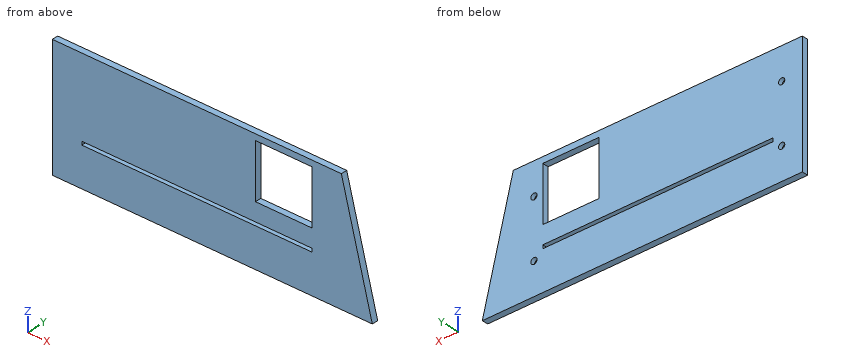
from build123d import *

# Parameters (mm, degrees)
F0_W     = 140
F0_H     = 59
F1_DEPTH = 3
F2_W     = 111.440674
F2_H     = 1.685995
F3_DEPTH = 25
F4_W     = 27.34
F4_H     = 19
F5_DEPTH = 25
F6_R     = 1.5
F7_DEPTH = 2
F8_W     = 27.34
F8_H     = 26.557377
F9_DEPTH = 25


with BuildPart() as f1:
    # F0 (on Front) → F1 (new body)
    with BuildSketch(Plane.XZ):
        Rectangle(F0_W, F0_H)
        Polygon((85, -29.5), (70, 29.5), (70, -29.5), align=None)
    extrude(amount=F1_DEPTH)

    # F2 (on face) → F3 (cut)
    with BuildSketch(Plane.XZ.offset(3)):
        with Locations((0, -9.62422)):
            Rectangle(F2_W, F2_H)
    extrude(amount=-F3_DEPTH, mode=Mode.SUBTRACT)

    # F4 (on face) → F5 (cut)
    with BuildSketch(Plane.XZ.offset(3)):
        with Locations((42.050337, 12.718777)):
            Rectangle(F4_W, F4_H)
    extrude(amount=-F5_DEPTH, mode=Mode.SUBTRACT)

    # F6 (on face) → F7 (cut)
    with BuildSketch(Plane(origin=(0, 0, 0), x_dir=(-1, 0, 0), z_dir=(0, 1, 0))):
        with Locations((60, 14)):
            Circle(F6_R)
        with Locations((-60, 14)):
            Circle(F6_R)
        with Locations((60, -14)):
            Circle(F6_R)
        with Locations((-60, -14)):
            Circle(F6_R)
    extrude(amount=-F7_DEPTH, mode=Mode.SUBTRACT)

    # F8 (on face) → F9 (cut)
    with BuildSketch(Plane.XZ.offset(3)):
        with Locations((42.050337, 13.278688)):
            Rectangle(F8_W, F8_H)
    extrude(amount=-F9_DEPTH, mode=Mode.SUBTRACT)


solid = f1.part
Source: CAD feature listing. Evaluate the final solid. Frame: model axes, mm. Round coordinates to 2 decimals unless told otherwise and drop trailing zeros. Order: outer loops, then holes, each group sorted by start corner. A loop starts at its lowest first (then second) coordinate and runs counter-clockwise, first axis right, second up. Notation, with made-up numbers: (26.25, 33.25) - (59.25, 33.25) arc R27 ccw to (59.25, 69.25) - close; hole circle Ø4 at (17, -13). An arc over 180 degrees is marked (long way). Use a Markdown table: item, result. Add a question column.
1. Section query A-A (x = 39). Return the cut outline in (y, z).
2. Section query D-D (z = 14). Return the cut outline in (x, y).
3. Line query: probe 1 along Z at (x, y) = (60, -0.5); probe 2 along Z at (x, y) = (34, -2.1); probe 3 along Z at (x, y) = (13, -2.45). Output: solid intervals per line, ascending.
4. Section query C-C (x = -32). Return the cut outline in (y, z), then the cut area to 3 significant figures.
5. First-contact query: pin 1 (5 mm diameter, centred on x = 1, z = -18.5, fed in from +Y); pin 2 (0.5 mm diameter, centred on y = -2, z = -9.5, fed in from +X); pin 3 (1.5 mm diameter, centred on y = -2, z = 8.5, fed in from +X); pin 4 (0.9 mm diameter, centred on x = -60.5, z = -14.5, fed in from +Y). Flat tips, straight axial feed; report the tip coordinate or a pass-through.
6. Section query B-B (y = -0.85). Return the cut outline in (x, z).
Derived:
| question | item | result |
|---|---|---|
| 1 | outline | (-3, -29.5) - (0, -29.5) - (0, -10.47) - (-3, -10.47) - close; (-3, -8.78) - (0, -8.78) - (0, 0) - (-3, 0) - close; (-3, 26.56) - (0, 26.56) - (0, 29.5) - (-3, 29.5) - close |
| 2 | outline | (-70, -3) - (28.38, -3) - (28.38, 0) - (-58.5, 0) - (-58.5, -2) - (-61.5, -2) - (-61.5, 0) - (-70, 0) - close; (55.72, -3) - (73.94, -3) - (73.94, 0) - (61.5, 0) - (61.5, -2) - (58.5, -2) - (58.5, 0) - (55.72, 0) - close |
| 3 | probe 1 | -29.5 to -15.5, -12.5 to 12.5, 15.5 to 29.5 |
| 3 | probe 2 | -29.5 to -10.47, -8.78 to 0, 26.56 to 29.5 |
| 3 | probe 3 | -29.5 to -10.47, -8.78 to 29.5 |
| 4 | outline | (-3, -29.5) - (0, -29.5) - (0, -10.47) - (-3, -10.47) - close; (-3, -8.78) - (0, -8.78) - (0, 29.5) - (-3, 29.5) - close |
| 4 | area | 172 mm2 |
| 5 | pin 1 | y = 0 |
| 5 | pin 2 | x = 79.98 |
| 5 | pin 3 | x = 75.53 |
| 5 | pin 4 | y = -2 |
| 6 | outline | (-70, -29.5) - (85, -29.5) - (70, 29.5) - (-70, 29.5) - close; hole circle Ø3 at (-60, -14); hole circle Ø3 at (-60, 14); hole (-55.72, -10.47) - (55.72, -10.47) - (55.72, -8.78) - (-55.72, -8.78) - close; hole (28.38, 0) - (55.72, 0) - (55.72, 26.56) - (28.38, 26.56) - close; hole circle Ø3 at (60, -14); hole circle Ø3 at (60, 14) |
